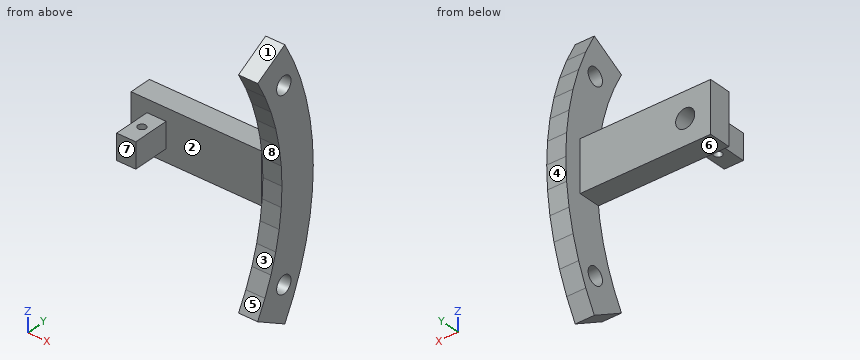
```python
from build123d import *

# Parameters (mm, degrees)
FOOT_DEPTH                     = 6
RISER_SKETCH_W                 = 41
RISER_SKETCH_H                 = 7
RISER_DEPTH                    = 8
TAB_SKETCH_W                   = 6
TAB_SKETCH_H                   = 11.6
PUSHROD_TAB_DEPTH              = 4
PIN_HOLE_SKETCH_W              = 3
PIN_HOLE_SKETCH_H              = 7
BALL_JOINT_HOLE_SKETCH_R       = 1.25
BALL_JOINT_HOLE_DEPTH          = 5
FOOT_BOLT_HOLE_22_5_SKETCH_R   = 2.75
FOOT_BOLT_HOLE_22_5_DEPTH      = 6
FOOT_BOLT_HOLE_22_5_SKETCH_2_R = 2.75
FOOT_BOLT_HOLE_22_5_2_DEPTH    = 6


with BuildPart() as part:
    # Foot Sketch → Foot (new body)
    with BuildSketch(Plane(origin=(-9, 0, 0), x_dir=(0, 0, -1), z_dir=(1, 0, 0))):
        Polygon((-40.75, 70.581070408), (-34.443388332, 73.864084643), (-27.874641681, 76.584948594), (-21.093752176, 78.722954843), (-14.15232648, 80.26183187), (-7.103193034, 81.189867894), (0, 81.5), (7.103193034, 81.189867894), (14.15232648, 80.26183187), (21.093752176, 78.722954843), (27.874641681, 76.584948594), (34.443388332, 73.864084643), (40.75, 70.581070408), (34.75, 60.188765563), (29.371969191, 62.988391199), (23.770399961, 65.308637145), (17.987923635, 67.131844927), (12.068548348, 68.444138834), (6.057324121, 69.235531517), (0, 69.5), (-6.057324121, 69.235531517), (-12.068548348, 68.444138834), (-17.987923635, 67.131844927), (-23.770399961, 65.308637145), (-29.371969191, 62.988391199), (-34.75, 60.188765563), align=None)
    extrude(amount=-FOOT_DEPTH)

    # Riser Sketch → Riser (add, symmetric)
    with BuildSketch(Plane.XY):
        with Locations((-35.5, 72.5)):
            Rectangle(RISER_SKETCH_W, RISER_SKETCH_H)
    extrude(amount=RISER_DEPTH, both=True)

    # Tab Sketch → Pushrod Tab (add, symmetric)
    with BuildSketch(Plane.XY):
        with Locations((-48, 63.2)):
            Rectangle(TAB_SKETCH_W, TAB_SKETCH_H)
    extrude(amount=PUSHROD_TAB_DEPTH, both=True)

    # Pin Hole Sketch → Pin Hole (revolve, cut)
    with BuildSketch(Plane.XY, mode=Mode.PRIVATE) as pin_hole_sk:
        with Locations((-46.5, 73.5)):
            Rectangle(PIN_HOLE_SKETCH_W, PIN_HOLE_SKETCH_H)
    revolve(pin_hole_sk.sketch.rotate(Axis((-48, 59, 0), (0, 1, 0)), 90), axis=Axis((-48, 59, 0), (0, 1, 0)), mode=Mode.SUBTRACT)

    # Ball Joint Hole Sketch → Ball Joint Hole (cut, symmetric)
    with BuildSketch(Plane.XY):
        with Locations((-48, 63.4)):
            Circle(BALL_JOINT_HOLE_SKETCH_R)
    extrude(amount=BALL_JOINT_HOLE_DEPTH, both=True, mode=Mode.SUBTRACT)

    # Foot Bolt Hole _22.5 Sketch → Foot Bolt Hole _22.5 (cut)
    with BuildSketch(Plane(origin=(-9, 0, 0), x_dir=(0, 0, -1), z_dir=(1, 0, 0))):
        with Locations((29.08394086, 70.214844471)):
            Circle(FOOT_BOLT_HOLE_22_5_SKETCH_R)
    extrude(amount=-FOOT_BOLT_HOLE_22_5_DEPTH, mode=Mode.SUBTRACT)

    # Foot Bolt Hole -22.5 Sketch 2 → Foot Bolt Hole -22.5 2 (cut)
    with BuildSketch(Plane(origin=(-9, 0, 0), x_dir=(0, 0, -1), z_dir=(1, 0, 0))):
        with Locations((-29.08394086, 70.214844471)):
            Circle(FOOT_BOLT_HOLE_22_5_SKETCH_2_R)
    extrude(amount=-FOOT_BOLT_HOLE_22_5_2_DEPTH, mode=Mode.SUBTRACT)


solid = part.part
```
Work out the finished part from the listing and answer in its coordinate system (mm). Face numbers are marked on the shaded views. A direction names the side the tool comes from. Give positions to 0.01 mm unless a question says otherwise; leave off trailing zeros. Loops run counter-clockwise (first coordinate to the right, second up) from the corner with the lowest first, then second, coordinate; pieces in that order, holes last. Notation, with made-up numbers: (22.25, 51.25) -> (76.25, 51.25) arc R28 cw to (76.25, 76.25) -> close; hole circle Ø3 at (68, 55.25). An arc over 180 degrees is marked (long way). Use CSV: the item, a comma, the result in double quotes.
1. Flat-ended cylindrical pins translate along their axes: pin 1 Ø1.8 at (x, z) = (-47, 1.5) entering from +Y; pin 2 Ø2 at (x, y) = (-34, 75.5) entering from -Z; pin 3 Ø17.5 at (x, z) = (-26.5, -2) entering from +Y; pin 4 Ø12 at (y, z) = (65.5, 4.5) entering from -X. Find the tip coordinate at first contact, or state that the pin passes through.
Found:
pin 1,"y = 70"
pin 2,"z = -8"
pin 3,"y = 76"
pin 4,"x = -56"
2. The mould has two halves that part along Z. Classify the marked faces 1, 2, 3 and 4: +Z half, -Z half, draft (parallel to the pull), parting line (faces both ways), or undercut.
Found:
face 1,"+Z half"
face 2,"draft"
face 3,"undercut"
face 4,"-Z half"
3. The part is cut by section A-A (x = -48). Write down the section's boundary in (y, z).
Found:
outline,"(57.4, -4) -> (62.15, -4) -> (62.15, 4) -> (57.4, 4) -> close; (64.65, -4) -> (69, -4) -> (69, -8) -> (76, -8) -> (76, -3) -> (70, -3) -> (70, 3) -> (76, 3) -> (76, 8) -> (69, 8) -> (69, 4) -> (64.65, 4) -> close"
4. The part is cut by section B-B (y = 75). Write down the section's boundary in (x, z).
Found:
outline,"(-56, -8) -> (-15, -8) -> (-15, -31.7) -> (-9, -31.7) -> (-9, 31.7) -> (-15, 31.7) -> (-15, 8) -> (-56, 8) -> close; hole circle Ø6 at (-48, 0)"
5. Straight lines are drawn through the part: line 1 (X direction, y = 74.2, z = 0); line 2 (Z direction, x = -48, y = 72.2); line 3 (X direction, y = 73.25, z = 9.5). For each, find the intervals that lie inside material, in ascending order.
Found:
line 1,"-56 to -51, -45 to -9"
line 2,"-8 to -3, 3 to 8"
line 3,"-15 to -9"
6. A tool of negligible diameter and unlimited length cuts with its end or side. For the marked faces 5, 6, 7 and 8, from which of +Z, -Z, +X, -X, +Y, -Y can it reach the whole face along a straight path? Write none if from no direction.
Found:
face 5,"+X, -X, -Y"
face 6,"-Z, -X, +Y, -Y"
face 7,"+Z, -Z, +X, -X, -Y"
face 8,"+X, -Y"
7. The part is cut by section C-C (x = -39). Write down the section's boundary in (y, z), then the cut area to 3 significant figures.
Found:
outline,"(69, -8) -> (76, -8) -> (76, 8) -> (69, 8) -> close"
area,"112 mm^2"
8. The part is cut by section D-D (y = 59.25). Write down the section's boundary in (x, z).
Found:
outline,"(-51, -4) -> (-45, -4) -> (-45, 4) -> (-51, 4) -> close"
